from build123d import *

# Parameters (mm, degrees)
SKETCH1_R           = 7.5
SKETCH1_R_2         = 4.75
BOSS_EXTRUDE1_DEPTH = 8.35
BOSS_EXTRUDE2_DEPTH = 3.35
BOSS_EXTRUDE3_START = 8.35
SKETCH1_4_R         = 4.75
BOSS_EXTRUDE3_DEPTH = 7


with BuildPart() as part:
    # Sketch1 → Boss-Extrude1 (new body)
    with BuildSketch(Plane.XY):
        Circle(SKETCH1_R)
        Polygon((-3.290896534, 5.7), (-6.581793069, 0), (-3.290896534, -5.7), (3.290896534, -5.7), (6.581793069, 0), (3.290896534, 5.7), align=None, mode=Mode.SUBTRACT)
        Circle(SKETCH1_R)
        Circle(SKETCH1_R_2, mode=Mode.SUBTRACT)
        Circle(SKETCH1_R_2)
    extrude(amount=BOSS_EXTRUDE1_DEPTH)

    # Sketch1<3> → Boss-Extrude2 (add)
    with BuildSketch(Plane.XY):
        Polygon((-3.290896534, -5.7), (3.290896534, -5.7), (6.581793069, 0), (3.290896534, 5.7), (-3.290896534, 5.7), (-6.581793069, 0), align=None)
    extrude(amount=-BOSS_EXTRUDE2_DEPTH)

    # Sketch1<4> → Boss-Extrude3 (add)
    with BuildSketch(Plane.XY.offset(BOSS_EXTRUDE3_START)):
        Circle(SKETCH1_4_R)
    extrude(amount=BOSS_EXTRUDE3_DEPTH)


solid = part.part
Check sheet for the modelled part. Datum: model origin and axes. Units: mm. A direction names the side the tool comes from. Give positions to 0.01 mm unless a question says otherwise; leave off trailing zeros. Loops run counter-clockwise (first coordinate to the right, second up) from the corner with the lowest first, then second, coordinate; pieces in that order, holes last. Notation, with made-up numbers: M 73,-23 L 101,-23 A24 ccw 101,14 Z; hole C -1.5,63 d7. An arc over 180 degrees is marked long. Answer as a JSON object with one key per item and string values. Group by question number.
Q1. Cross-section at C-C on z = -2. Record the cut outline in (x, y).
Q2. Go/stop test with flat-tipped pins: P1, Ø1, axis at x = 0.5, z = -2, coming from the -Y side; P2, Ø4, axis at x = 6, z = 11.5, coming from the +Y side; P3, Ø1.5, axis at x = 3, z = 9, coming from the -Y side. Record where each tip stops, or that it passes through.
Q3. Release check for a two-part mould opening along Z. For faces 6 (the flat face through (0, -5, 8.35)), 7 (the flat face through (0, 0, -3.35)), 8 (the cylindrical face through (-7.493, 0.33, 4.117)) record: released by +Z, released by -Z, zero draft, split by the parting line, or undercut.
Q4. Material ranges on line 1 along Z through (x, y) = (3.5, -3.5); line 2 along Z through (x, y) = (-6, 2.75); line 3 along Y through (x, z) = (-0.75, -0.25), recorded low to high. Write a range as [from, to].
Q5. Access from +Z, -Z, +X, -X, +Y, -Y to the whole of each face (thin tool, end or side, straight path). Record for faces 1 (the flat face through (0, -6, 0)), 2 (the flat face through (0, -5.7, -2)), 3 (the cylindrical face through (2.192, -4.214, 11.801)), 4 (the flat face through (0, 5.7, -2)), 5 (the flat face through (4.913, -2.89, -1.652)).
Q6. Cross-section at D-D on y = -6. Record the cut outline in (x, z), then the cut area to 4 significant figures.
Q7. Cross-section at A-A on x = 0. Record the cut outline in (y, z), then the cut area to 3 significant figures.
Q8. Cross-section at B-B on y = 4.5. Record the cut outline in (x, z).
Evaluation:
{
 "1": {"outline": "M -6.58,0 L -3.29,-5.7 L 3.29,-5.7 L 6.58,0 L 3.29,5.7 L -3.29,5.7 Z"},
 "2": {"P1": "stops at y = -5.7", "P2": "stops at y = 2.56", "P3": "stops at y = -7.03"},
 "3": {"face 6": "released by +Z", "face 7": "released by -Z", "face 8": "zero draft"},
 "4": {"line 1": "z = [-3.35, 8.35]", "line 2": "z = [0, 8.35]", "line 3": "y = [-5.7, 5.7]"},
 "5": {"face 1": "-Z", "face 2": "-Z, +X, -X, -Y", "face 3": "+Z", "face 4": "-Z, +X, -X, +Y", "face 5": "-Z, +X, -Y"},
 "6": {"outline": "M -4.5,0 L 4.5,0 L 4.5,8.35 L -4.5,8.35 Z", "area": "75.15 mm2"},
 "7": {"outline": "M -7.5,0 L -5.7,0 L -5.7,-3.35 L 5.7,-3.35 L 5.7,0 L 7.5,0 L 7.5,8.35 L 4.75,8.35 L 4.75,15.35 L -4.75,15.35 L -4.75,8.35 L -7.5,8.35 Z", "area": "230 mm2"},
 "8": {"outline": "M -6,0 L -3.98,0 L -3.98,-3.35 L 3.98,-3.35 L 3.98,0 L 6,0 L 6,8.35 L 1.52,8.35 L 1.52,15.35 L -1.52,15.35 L -1.52,8.35 L -6,8.35 Z"}
}
